The listing builds one solid part. Answer for the finished solid, in the listing's coordinates (mm). A direction names the side the tool comes from. Give positions to 0.01 mm unless a question says otherwise; leave off trailing zeros. Write each loop counter-clockwise with the first axis right and the second up, starting at its lowest first coordinate (ties: lowest second). Pieces come first, ordered by that corner, then holes. Notation, with made-up numbers: (-3, 3.5) - (34, 3.5) arc R29 cw to (34, 36.5) - close; hole circle Ø6 at (51, 42.5). An arc over 180 degrees is marked (long way). Answer as CSV lines item,"result". Start each with the question number.
(1) For faces 1 (the face through (7.213, -14, -5)), 2 (the face through (15, -15, -6.35)), 3 (the face through (24, -15, 0)), 4 (the face through (9, -10.565, -3)), determine the directions among +Z, -Z, +X, -X, +Y, -Y from which every point of the face is accessible in a straight line to the end or side of a thin tool.
(2) Find section C-C (z = 1). State how many separate pieces and enclosed holes the cut face has, then the cut area to 3 significant figures.
(3) Find section A-A (z = -5.5). Write down the section's boundary in (x, y).
(4) Find section B-B (x = 18). Write down the section's boundary in (y, z) (3 decimals).
(5) For a pull along Z with two mould halves and no side action, classify faces 5 (the face through (13.763, -14, -5)), 6 (the face through (9, -15, -6.35)), 7 (the face through (15.328, -16.992, -3.519)), 8 (the face through (8.778, -16.992, -3.519)) as pulls with the +Z half, pulls with the -Z half, needs draft (parallel to the pull), parting line crosses it, or undercut.
(6) Each of these flat-tipped pins is pushed along its axis until it touches: pin 1 Ø1.5 at (y, z) = (-15, -1) entering from -X; pin 2 Ø1.9 at (y, z) = (-15.44, -3.18) entering from -X; pin 3 Ø3 at (x, y) = (27.94, -15.24) entering from -Z; pin 4 Ø3 at (y, z) = (-13.5, -2) entering from +X. Where does it stop, or does it pass through?
(7) Straight lines are drawn through the part: probe 1 along X at (y, z) = (-18, -0.25); probe 2 along X at (y, z) = (-15.24, 2.05); probe 3 along X at (y, z) = (-14.5, 1.5). For each, find the intervals that lie inside material, in ascending order.
Autodesk Inventor part; units mm, degrees
ref_plane "YZ Plane" through (0, 0, 0) normal (1, 0, 0) x (0, 1, 0)
ref_plane "XZ Plane" through (0, 0, 0) normal (0, 1, 0) x (-1, 0, 0)
ref_plane "XY Plane" through (0, 0, 0) normal (0, 0, 1) x (1, 0, 0)
ref_plane "Work Plane1" through (0, 0, 0) normal (0, 0, 1) x (1, 0, 0)
sketch "Sketch1" plane through (0, 0, 0) normal (0, 0, 1) x (1, 0, 0)
  line L0 (31.75, -13.716) -> (31.75, -6.096)
  arc A0 (25.146, -20.32) -> (31.75, -13.716) centre (25.146, -13.716) ccw
  line L1 (24.13, -20.32) -> (25.146, -20.32)
  circle A1 centre (27.94, -15.24) radius 1.1303
  line L2 (31.75, -6.096) -> (31.75, -10.4198)
  line L3 (31.75, -10.4198) -> (24.13, -10.4198)
  line L4 (24.13, -10.4198) -> (24.13, -20.32)
  point P0 (0, 0)
extrude "Extrusion1" add sketch "Sketch1" along normal blind 3.175
move faces "Move1" translate (-20.6502, 0, 0) faces at (24.13, -13.7199, 1.0583)
sketch "Sketch2" plane through (0, 0, 0) normal (0, 0, -1) x (-1, 0, 0)
  line L0 (-13.6627, -7.7169) -> (-13.6627, -20.1208)
  line L1 (-10.4877, -7.7169) -> (-10.4877, -20.1208)
  line L2 (-3.4798, -20.32) -> (-25.146, -20.32)
  line L3 (-10.3877, -20.32) -> (-7.2127, -20.32)
  line L4 (-7.2127, -20.32) -> (-7.2127, -10.5651)
  line L5 (-7.2127, -10.5651) -> (-10.3877, -10.5651)
  line L6 (-10.3877, -10.5651) -> (-10.3877, -20.32)
  line L7 (-31.75, -10.4198) -> (-3.4798, -10.4198)
  line L8 (-13.7627, -20.32) -> (-16.9377, -20.32)
  line L9 (-16.9377, -20.32) -> (-16.9377, -10.4198)
  line L10 (-16.9377, -10.4198) -> (-13.7627, -10.4198)
  line L11 (-13.7627, -10.4198) -> (-13.7627, -20.32)
  point P0 (0, 0)
  dimension "d5" = 0.1
  dimension "d6" = 0.1
  dimension "d7" = 3.175
  dimension "d8" = 3.175
extrude "Extrusion2" add sketch "Sketch2" along normal blind 6.35
sketch "Sketch3" plane through (6.6139, -20.32, 0) normal (-1, 0, 0) x (0, 0, 1)
  line L0 (0, 9.7549) -> (0, 0) construction
  line L1 (0, 9.7549) -> (-6.35, 9.7549) construction
  line L2 (-6.35, 0) -> (-6.35, 9.7549) construction
  line L3 (0, 0) -> (-6.35, 0) construction
  line L4 (0, 0) -> (-6.35, 9.7549) construction
  circle A0 centre (-3.175, 4.8775) radius 1.5875
  point P0 (0, 20.32)
  dimension "d11" = 3.175
extrude "Extrusion3" [suppressed]
sketch "Sketch4" plane through (0, 0, 0) normal (0, 0, -1) x (-1, 0, 0)
  line L0 (-16.9377, -20.32) -> (-16.9377, -10.4198) construction
  line L1 (-16.9377, -15.3699) -> (-22.7751, -15.3699) construction
  circle A0 centre (-18.5252, -15.3699) radius 1.5875
  point P0 (0, 0)
  dimension "d17" = 3.175
extrude "Extrusion4" cut sketch "Sketch4" against normal blind 12.7
sketch "Sketch5" plane through (7.2127, -20.32, 0) normal (-1, 0, 0) x (0, 0, 1)
  line L0 (0, 9.7549) -> (0, 0)
  line L1 (-6.35, 0) -> (-6.35, 9.7549)
  line L2 (0, 9.7549) -> (-6.35, 0) construction
  circle A0 centre (-3.175, 4.8775) radius 1.5875
  point P0 (0, 20.32)
  dimension "d20" = 3.175
extrude "Extrusion5" cut sketch "Sketch5" against normal blind 17.4625
properties part number "adapter_1"
Result set:
1,face 1,"-Z, -X, +Y, -Y"
1,face 2,"-Z, +X, -X, +Y, -Y"
1,face 3,"-Z, +X, +Y, -Y"
1,face 4,"-Z, -X, +Y"
2,separate pieces,"1"
2,enclosed holes,"2"
2,area,"259 mm^2"
3,outline,"(7.21, -20.32) - (10.39, -20.32) - (10.39, -10.57) - (7.21, -10.57) - close; (13.76, -20.32) - (16.94, -20.32) - (16.94, -10.42) - (13.76, -10.42) - close"
4,outline,"(-20.32, 0) - (-16.868, 0) - (-16.868, 3.175) - (-20.32, 3.175) - close; (-13.872, 0) - (-10.42, 0) - (-10.42, 3.175) - (-13.872, 3.175) - close"
5,face 5,"needs draft"
5,face 6,"pulls with the -Z half"
5,face 7,"undercut"
5,face 8,"undercut"
6,pin 1,"x = 7.21"
6,pin 2,"through"
6,pin 3,"z = 0"
6,pin 4,"x = 16.94"
7,probe 1,"7.21 to 10.39, 13.76 to 16.94"
7,probe 2,"3.48 to 16.94, 20.11 to 26.81, 29.07 to 31.57"
7,probe 3,"3.48 to 17.2, 19.85 to 27.09, 28.79 to 31.7"
